```python
from build123d import *

# Parameters (mm, degrees)
CROQUIS1_W                = 620
CROQUIS1_H                = 200
CROQUIS1_W_2              = 534
CROQUIS1_H_2              = 114
SALIENTE_EXTRUIR1_DEPTH   = 6
CROQUIS2_W                = 6.02
CROQUIS2_H                = 40
CORTAR_EXTRUIR1_DEPTH     = 6
CROQUIS3_W                = 40
CROQUIS3_H                = 6.02
CORTAR_EXTRUIR2_DEPTH     = 6
MATRIZL1_COUNT            = 6
MATRIZL1_PITCH            = 80
SIMETR_A1_COPY_1_SKETCH_W = 40
SIMETR_A1_COPY_1_SKETCH_H = 6.02
SIMETR_A1_COPY_1_DEPTH    = 6
SIMETR_A1_COPY_2_SKETCH_W = 40
SIMETR_A1_COPY_2_SKETCH_H = 6.02
SIMETR_A1_COPY_2_DEPTH    = 6
SIMETR_A1_COPY_3_SKETCH_W = 40
SIMETR_A1_COPY_3_SKETCH_H = 6.02
SIMETR_A1_COPY_3_DEPTH    = 6
SIMETR_A1_COPY_4_SKETCH_W = 40
SIMETR_A1_COPY_4_SKETCH_H = 6.02
SIMETR_A1_COPY_4_DEPTH    = 6
SIMETR_A1_COPY_5_SKETCH_W = 40
SIMETR_A1_COPY_5_SKETCH_H = 6.02
SIMETR_A1_COPY_5_DEPTH    = 6


with BuildPart() as part:
    # Croquis1 → Saliente-Extruir1 (new body)
    with BuildSketch(Plane.XY):
        Rectangle(CROQUIS1_W, CROQUIS1_H)
        Rectangle(CROQUIS1_W_2, CROQUIS1_H_2, mode=Mode.SUBTRACT)
    extrude(amount=SALIENTE_EXTRUIR1_DEPTH)

    # Croquis2 → Cortar-Extruir1 (cut)
    with BuildSketch(Plane.XY.offset(6)):
        with Locations((-275.01, 40)):
            Rectangle(CROQUIS2_W, CROQUIS2_H)
        with Locations((-275.01, -40)):
            Rectangle(CROQUIS2_W, CROQUIS2_H)
        with Locations((275.01, -40)):
            Rectangle(CROQUIS2_W, CROQUIS2_H)
        with Locations((275.01, 40)):
            Rectangle(CROQUIS2_W, CROQUIS2_H)
    extrude(amount=-CORTAR_EXTRUIR1_DEPTH, mode=Mode.SUBTRACT)

    # Croquis3 → Cortar-Extruir2 (cut)
    with BuildSketch(Plane.XY.offset(6)):
        with Locations((-212, 64.01)):
            Rectangle(CROQUIS3_W, CROQUIS3_H)
    cortar_extruir2 = extrude(amount=-CORTAR_EXTRUIR2_DEPTH, mode=Mode.SUBTRACT)

    # MatrizL1: Cortar-Extruir2 ×6
    with Locations(*[(i * MATRIZL1_PITCH, 0, 0) for i in range(1, MATRIZL1_COUNT)]):
        add(cortar_extruir2, mode=Mode.SUBTRACT)

    # Simetría1: Cortar-Extruir2 across plane
    add(cortar_extruir2.mirror(Plane.ZX), mode=Mode.SUBTRACT)

    # Simetría1 copy 1 sketch → Simetría1 copy 1 (cut)
    with BuildSketch(Plane(origin=(80, 0, 6), x_dir=(1, 0, 0), z_dir=(0, 0, 1))):
        with Locations((-212, -64.01)):
            Rectangle(SIMETR_A1_COPY_1_SKETCH_W, SIMETR_A1_COPY_1_SKETCH_H)
    extrude(amount=-SIMETR_A1_COPY_1_DEPTH, mode=Mode.SUBTRACT)

    # Simetría1 copy 2 sketch → Simetría1 copy 2 (cut)
    with BuildSketch(Plane(origin=(160, 0, 6), x_dir=(1, 0, 0), z_dir=(0, 0, 1))):
        with Locations((-212, -64.01)):
            Rectangle(SIMETR_A1_COPY_2_SKETCH_W, SIMETR_A1_COPY_2_SKETCH_H)
    extrude(amount=-SIMETR_A1_COPY_2_DEPTH, mode=Mode.SUBTRACT)

    # Simetría1 copy 3 sketch → Simetría1 copy 3 (cut)
    with BuildSketch(Plane(origin=(240, 0, 6), x_dir=(1, 0, 0), z_dir=(0, 0, 1))):
        with Locations((-212, -64.01)):
            Rectangle(SIMETR_A1_COPY_3_SKETCH_W, SIMETR_A1_COPY_3_SKETCH_H)
    extrude(amount=-SIMETR_A1_COPY_3_DEPTH, mode=Mode.SUBTRACT)

    # Simetría1 copy 4 sketch → Simetría1 copy 4 (cut)
    with BuildSketch(Plane(origin=(320, 0, 6), x_dir=(1, 0, 0), z_dir=(0, 0, 1))):
        with Locations((-212, -64.01)):
            Rectangle(SIMETR_A1_COPY_4_SKETCH_W, SIMETR_A1_COPY_4_SKETCH_H)
    extrude(amount=-SIMETR_A1_COPY_4_DEPTH, mode=Mode.SUBTRACT)

    # Simetría1 copy 5 sketch → Simetría1 copy 5 (cut)
    with BuildSketch(Plane(origin=(400, 0, 6), x_dir=(1, 0, 0), z_dir=(0, 0, 1))):
        with Locations((-212, -64.01)):
            Rectangle(SIMETR_A1_COPY_5_SKETCH_W, SIMETR_A1_COPY_5_SKETCH_H)
    extrude(amount=-SIMETR_A1_COPY_5_DEPTH, mode=Mode.SUBTRACT)


solid = part.part
```
Input: part model. Units: mm. Frame: model coordinates. Give positions to 0.01 mm unless a question says otherwise; leave off trailing zeros. Order: outer loops, then holes, each group sorted by start corner. A loop starts at its lowest first (then second) coordinate and runs counter-clockwise, first axis right, second up. Notation, with made-up numbers: M -11.5,-21 L 40.5,-21 A19 ccw 40.5,-2 Z; hole C -21.75,75 d3. An arc over 180 degrees is marked long. Return JSON: item names as keys, results as strings.
1) Section query C-C on x = -95. Output: boundary loops of the cut face in (y, z), and give its area (3 significant figures).
Taken from the geometry:
{"outline": "M -100,0 L -57,0 L -57,6 L -100,6 Z; M 57,0 L 100,0 L 100,6 L 57,6 Z", "area": "516 mm2"}
2) Section query A-A on y = 46. Output: boundary loops of the cut face in (x, z), and give its area (3 significant figures).
Taken from the geometry:
{"outline": "M -310,0 L -278.02,0 L -278.02,6 L -310,6 Z; M -272,0 L -267,0 L -267,6 L -272,6 Z; M 267,0 L 272,0 L 272,6 L 267,6 Z; M 278.02,0 L 310,0 L 310,6 L 278.02,6 Z", "area": "444 mm2"}
3) Contact query for a flat-ended pin moving along its axis: pin 1 (2 mm diameter, centred on x = 136.5, y = -79.5, fed in from -Z). Output: stop coordinate, or through.
Taken from the geometry:
{"pin 1": "stops at z = 0"}
4) Section query B-B on x = 175.5. Output: boundary loops of the cut face in (y, z).
Taken from the geometry:
{"outline": "M -100,0 L -67.02,0 L -67.02,6 L -100,6 Z; M -61,0 L -57,0 L -57,6 L -61,6 Z; M 57,0 L 61,0 L 61,6 L 57,6 Z; M 67.02,0 L 100,0 L 100,6 L 67.02,6 Z"}
5) Line query: L1, parallel to Y at x = -193, z = 4.7; L2, parallel to X at y = -54.5, z = 2.9; L3, parallel to Y at x = 272.5, z = 3.6. Output: solid intervals per line, ascending. Write a range as [from, to].
Taken from the geometry:
{"L1": "y = [-100, -67.02], [-61, -57], [57, 61], [67.02, 100]", "L2": "x = [-310, -278.02], [-272, -267], [267, 272], [278.02, 310]", "L3": "y = [-100, -60], [-20, 20], [60, 100]"}
6) Section query D-D on z = 2.5. Count the separate pieces of the cut face and the enclosed holes in it, and give its area (3 significant figures).
Taken from the geometry:
{"separate pieces": "1", "enclosed holes": "17", "area": "59,300 mm2"}
